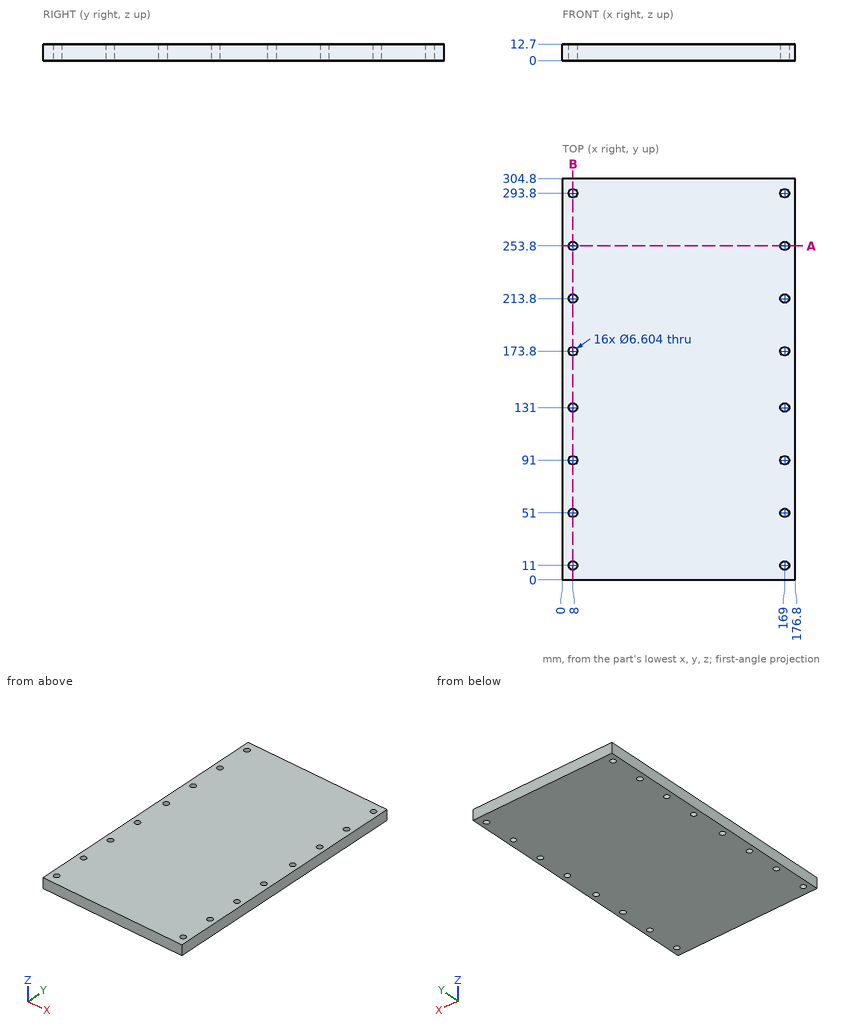
The drawing under review shows one solid part. Ordinate dimensions are in mm from its lowest x, y, z. Coordinates: 2 decimals unless noted, no trailing zeros. Loops run counter-clockwise (first coordinate to the right, second up) from the corner with the lowest first, then second, coordinate; pieces in that order, holes last.
Item 1: Add section A-A (y = 253.8). Write out the cut boundary in (x, z), and give its area (3 significant figures).
Completed:
outline: (0, 0) - (4.7, 0) - (4.7, 12.7) - (0, 12.7) - close; (11.3, 0) - (165.7, 0) - (165.7, 12.7) - (11.3, 12.7) - close; (172.3, 0) - (176.8, 0) - (176.8, 12.7) - (172.3, 12.7) - close
area: 2,080 mm2
Item 2: Wall thickness on L1, parallel to X at y = 51, z = 4.75: over which ranges is the line inside the solid? List them lowest first.
Completed:
L1: x = 0 to 4.7, 11.3 to 165.7, 172.3 to 176.8
Item 3: Clearance check with a flat-ended pin moving along its axis: pin 1 (4 mm diameter, centred on x = 8, y = 173.8, fed in from +Z). State where the tip first meets the part, or that it passes through.
Completed:
pin 1: passes through
Item 4: Add section B-B (x = 8). Give the number of separate pieces and of enclosed holes in the cut face, and give its area (3 significant figures).
Completed:
separate pieces: 9
enclosed holes: 0
area: 3,200 mm2
